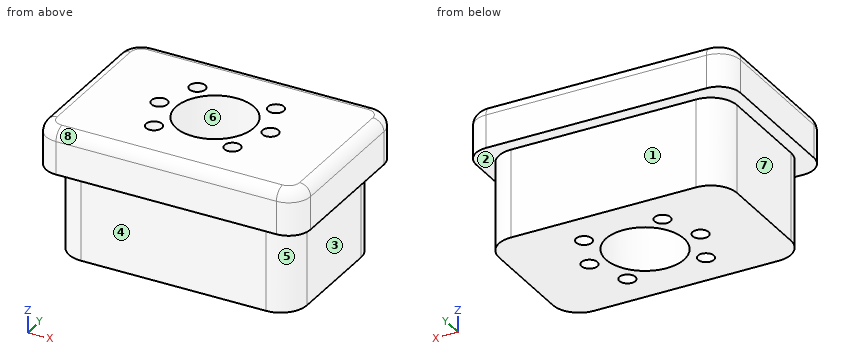
Autodesk Inventor part; units mm, degrees
ref_plane "YZ Plane" through (0, 0, 0) normal (1, 0, 0) x (0, 1, 0)
ref_plane "XZ Plane" through (0, 0, 0) normal (0, 1, 0) x (-1, 0, 0)
ref_plane "XY Plane" through (0, 0, 0) normal (0, 0, 1) x (1, 0, 0)
sketch "Sketch1" plane through (0, 0, 0) normal (0, 0, 1) x (1, 0, 0)
  line L0 (7.62, 0) -> (60.96, 0)
  line L1 (68.58, 7.62) -> (68.58, 35.56)
  line L2 (60.96, 43.18) -> (7.62, 43.18)
  line L3 (0, 35.56) -> (0, 7.62)
  arc A0 (7.62, 43.18) -> (0, 35.56) centre (7.62, 35.56) ccw
  arc A1 (0, 7.62) -> (7.62, 0) centre (7.62, 7.62) ccw
  arc A2 (68.58, 35.56) -> (60.96, 43.18) centre (60.96, 35.56) ccw
  arc A3 (60.96, 0) -> (68.58, 7.62) centre (60.96, 7.62) ccw
  point P0 (0, 0)
  point P1 (68.58, 43.18)
  point P2 (68.58, 0)
  point P3 (0, 43.18)
  dimension "d0" = 68.58
  dimension "d1" = 43.18
  dimension "d3" = 7.62
extrude "Extrusion1" add sketch "Sketch1" along normal blind 25.4
sketch "Sketch2" plane through (0, 0, 25.4) normal (0, 0, 1) x (1, 0, 0)
  line L0 (2.54, -3.81) -> (66.04, -3.81)
  line L1 (72.39, 2.54) -> (72.39, 40.64)
  line L2 (66.04, 46.99) -> (2.54, 46.99)
  line L3 (-3.81, 40.64) -> (-3.81, 2.54)
  line L4 (60.96, 43.18) -> (7.62, 43.18) construction
  line L5 (0, 35.56) -> (0, 7.62) construction
  line L6 (7.62, 0) -> (60.96, 0) construction
  line L7 (68.58, 7.62) -> (68.58, 35.56) construction
  arc A0 (2.54, 46.99) -> (-3.81, 40.64) centre (2.54, 40.64) ccw
  arc A1 (-3.81, 2.54) -> (2.54, -3.81) centre (2.54, 2.54) ccw
  arc A2 (66.04, -3.81) -> (72.39, 2.54) centre (66.04, 2.54) ccw
  arc A3 (72.39, 40.64) -> (66.04, 46.99) centre (66.04, 40.64) ccw
  point P0 (0, 0)
  point P1 (72.39, 46.99)
  point P2 (72.39, -3.81)
  point P3 (-3.81, 46.99)
  point P4 (34.29, 46.99)
  point P5 (34.29, 43.18)
  point P6 (68.58, 21.59)
  point P7 (72.39, 21.59)
  dimension "d6" = 76.2
  dimension "d7" = 50.8
  dimension "d8" = 6.35
extrude "Extrusion2" add sketch "Sketch2" along normal blind 12.7
fillet "Fillet1" radius 3.175 8 edges at (-1.9501, 45.1301, 38.1) (-3.81, 21.59, 38.1) (-1.9501, -1.9501, 38.1) (34.29, -3.81, 38.1) (70.5301, -1.9501, 38.1) (72.39, 21.59, 38.1) (70.5301, 45.1301, 38.1) (34.29, 46.99, 38.1)
sketch "Sketch3" plane through (0, 0, 38.1) normal (0, 0, 1) x (1, 0, 0)
  circle A0 centre (34.29, 21.59) radius 11.25
  line L0 (-0.635, 2.54) -> (-0.635, 40.64) construction
  line L1 (2.54, 43.815) -> (66.04, 43.815) construction
  circle A1 centre (34.29, 21.59) radius 16 construction
  circle A2 centre (45.6037, 32.9037) radius 2.3
  circle A3 centre (18.29, 21.59) radius 2.3
  circle A4 centre (45.6037, 10.2763) radius 2.3
  circle A5 centre (50.29, 21.59) radius 2.3
  circle A6 centre (22.9763, 32.9037) radius 2.3
  circle A7 centre (22.9763, 10.2763) radius 2.3
  line L2 (22.9763, 32.9037) -> (34.29, 21.59) construction
  line L3 (34.29, 21.59) -> (18.29, 21.59) construction
  point P0 (0, 0)
  point P1 (34.29, 43.815)
  point P2 (-0.635, 21.59)
  dimension "d12" = 22.5
  dimension "d13" = 32
  dimension "d14" = 4.6
  dimension "d15" = 45
extrude "Extrusion3" cut sketch "Sketch3" against normal up to surface (38.1 mm away)
properties part number "2x3_Spacer"
Build history of the part. All positions in model axes, mm. Face numbers are marked on the shaded views. A direction names the side the tool comes from. Round coordinates to 2 decimals unless told otherwise and drop trailing zeros. Loops run counter-clockwise (first coordinate to the right, second up) from the corner with the lowest first, then second, coordinate; pieces in that order, holes last.
Item 1: Two-plate mould, pull along X, no slides. Class the marked faces 6, 7 and 8: released by +X, released by -X, zero draft, split by the parting line, or undercut.
Item 2: Saw through at D-D (x = 21.5). List the corners of the cut face in (y, z) (3 decimals), then the cut area to 3 significant figures.
Item 3: Pin check, flat tips, straight feed: P1, Ø3, axis at x = 22.98, y = 32.9, coming from the -Z side (3 decimals); P2, Ø12.5, axis at x = 31, z = 17.5, coming from the -Y side; P3, Ø1, axis at y = 17.5, z = 21, coming from the -X side; P4, Ø7.5, axis at y = 21.5, z = 13, coming from the +X side. Stop position of each tip, or through.
Item 4: Saw through at A-A (x = 34.29). List the corners of the cut face in (y, z) (3 decimals), then the cut area to 3 significant figures.
Item 5: Saw through at B-B (y = 18). List the corners of the cut face in (x, z) (3 decimals), then the cut area to 3 significant figures.
Item 6: Which spindle directions (+Z, -Z, +X, -X, +Y, -Y) get a long thin tool onto all of the face, cutting with end or side? Do the marked faces 1, 2, 3, 4 and 5. Say none if no direction does.
Item 7: Drill centre lines: line 1 along Y through (x, z) = (47, 19); line 2 along X through (y, z) = (22, 20); line 3 along Y through (x, z) = (34, 15). Where is each one in solid material? Low to high.
Item 8: Saw through at C-C (z = 28). List the corners of the cut face in (x, y).
Worked answers:
1. face 6: undercut
1. face 7: released by -X
1. face 8: zero draft
2. outline: (-3.81, 25.4) - (0, 25.4) - (0, 0) - (8.513, 0) - (8.513, 38.1) - (-0.635, 38.1) arc R3.175 ccw to (-3.81, 34.925) - close; (12.04, 0) - (31.14, 0) - (31.14, 38.1) - (12.04, 38.1) - close; (34.667, 0) - (43.18, 0) - (43.18, 25.4) - (46.99, 25.4) - (46.99, 34.925) arc R3.175 ccw to (43.815, 38.1) - (34.667, 38.1) - close
2. area: 1,470 mm2
3. P1: passes through
3. P2: stops at y = 0
3. P3: stops at x = 0
3. P4: stops at x = 68.58
4. outline: (-3.81, 25.4) - (0, 25.4) - (0, 0) - (10.34, 0) - (10.34, 38.1) - (-0.635, 38.1) arc R3.175 ccw to (-3.81, 34.925) - close; (32.84, 0) - (43.18, 0) - (43.18, 25.4) - (46.99, 25.4) - (46.99, 34.925) arc R3.175 ccw to (43.815, 38.1) - (32.84, 38.1) - close
4. area: 880 mm2
5. outline: (-3.81, 25.4) - (0, 25.4) - (0, 0) - (23.628, 0) - (23.628, 38.1) - (-0.635, 38.1) arc R3.175 ccw to (-3.81, 34.925) - close; (44.952, 0) - (68.58, 0) - (68.58, 25.4) - (72.39, 25.4) - (72.39, 34.925) arc R3.175 ccw to (69.215, 38.1) - (44.952, 38.1) - close
5. area: 1,890 mm2
6. face 1: -Z, +X, -X, +Y
6. face 2: -Z
6. face 3: -Z, +X, +Y, -Y
6. face 4: -Z, +X, -X, -Y
6. face 5: -Z, +X, -Y
7. line 1: y = 0 to 8.45, 12.1 to 31.08, 34.73 to 43.18
7. line 2: x = 0 to 16.03, 20.55 to 23.05, 45.53 to 48.03, 52.55 to 68.58
7. line 3: y = 0 to 10.34, 32.84 to 43.18
8. outline: (-3.81, 2.54) arc R6.35 ccw to (2.54, -3.81) - (66.04, -3.81) arc R6.35 ccw to (72.39, 2.54) - (72.39, 40.64) arc R6.35 ccw to (66.04, 46.99) - (2.54, 46.99) arc R6.35 ccw to (-3.81, 40.64) - close; hole circle Ø4.6 at (18.29, 21.59); hole circle Ø4.6 at (22.98, 10.28); hole circle Ø4.6 at (22.98, 32.9); hole circle Ø22.5 at (34.29, 21.59); hole circle Ø4.6 at (45.6, 10.28); hole circle Ø4.6 at (45.6, 32.9); hole circle Ø4.6 at (50.29, 21.59)
